Read the model definition and answer for the solid it produces. Units are mm, in the model's axes. A direction names the side the tool comes from. Coordinates: 2 decimals unless noted, no trailing zeros. Loops run counter-clockwise (first coordinate to the right, second up) from the corner with the lowest first, then second, coordinate; pieces in that order, holes last.
Q1. Section D-D (z = 6.25) is taken. Give the vertices of the cut face in (x, y), then the cut area to 3 significant figures.
Q2. Section A-A (x = 0) is taken. Give the vertices of the cut face in (y, z).
Q3. Which of the six approach directions +Z, -Z, +X, -X, +Y, -Y give full straight-line access (tool end or side, diameter ignored) to faces 4 (the face through (0, 0, 5.6)), 5 (the face through (23.846, 7.509, 6.692))?
Q4. Straight lines are drawn through the part: line 1 (Y direction, x = 0, z = 4.5); line 2 (Y direction, x = 0, z = 9.5); line 3 (X direction, y = -0.5, z = 6.5) (3 decimals). For each, find the intervals that lie inside material, in ascending order.
Q5. Flat-ended cylindrical pins translate along their axes: P1, Ø5, axis at x = 8.5, z = 14.5, coming from the +Y side; P2, Ø1.5, axis at x = 19.5, z = 9.5, coming from the +Y side; P3, Ø6, axis at x = 11.5, z = 3.5, coming from the -Y side; P4, Ø10, axis at x = -20, y = 16.5, coming from the -Z side. Find the tip coordinate at first contact, or state that the pin passes through.
Q6. Section C-C (z = 15) is taken. Give the vertices of the cut face in (x, y), then the cut area to 3 significant figures.
Q7. The mould has two halves that part along X. Classify faces 1 (the face through (0, 0, -2)), 2 (the face through (-15, -13, 0)), 3 (the face through (-26.774, 1.178, 6.404)): pulls with the +X half, pulls with the -X half, needs draft (parallel to the pull), parting line crosses it, or undercut.
from build123d import *


with BuildPart() as part:
    # Sketch → Revolution (revolve)
    with BuildSketch(Plane.XZ):
        with BuildLine():
            Line((0, 5.6), (2.5, 5.6))
            Line((2.5, 5.6), (2.5, 2.6))
            Line((2.5, 2.6), (20.5, 2.6))
            Line((20.5, 2.6), (19.5, 0))
            Line((19.5, 0), (25, 0))
            Line((25, 0), (25, 13.2))
            ThreePointArc((25, 13.2), (24.598076, 14.7), (23.5, 15.798076))
            ThreePointArc((24.400016, 17.356913), (23.170591, 17.027501), (23.5, 15.798076))
            ThreePointArc((26.8, 13.2), (26.156926, 15.599992), (24.400016, 17.356913))
            Line((26.8, -0.585786), (26.8, 13.2))
            Line((25.385786, -2), (26.8, -0.585786))
            Line((0, -2), (25.385786, -2))
            Line((0, 5.6), (0, -2))
        make_face()
    revolve(axis=Axis((0, 0, 0), (0, 0, 1)))


solid = part.part
Numbers:
1. outline: circle Ø53.6 at (0, 0); hole circle Ø50 at (0, 0)
1. area: 293 mm2
2. outline: (-26.8, -0.59) - (-25.39, -2) - (25.39, -2) - (26.8, -0.59) - (26.8, 13.2) arc R4.8 ccw to (24.4, 17.36) arc R0.9 ccw to (23.5, 15.8) arc R3 cw to (25, 13.2) - (25, 0) - (19.5, 0) - (20.5, 2.6) - (2.5, 2.6) - (2.5, 5.6) - (-2.5, 5.6) - (-2.5, 2.6) - (-20.5, 2.6) - (-19.5, 0) - (-25, 0) - (-25, 13.2) arc R3 cw to (-23.5, 15.8) arc R0.9 ccw to (-24.4, 17.36) arc R4.8 ccw to (-26.8, 13.2) - close
3. face 4: +Z
3. face 5: none
4. line 1: y = -26.8 to -25, -2.5 to 2.5, 25 to 26.8
4. line 2: y = -26.8 to -25, 25 to 26.8
4. line 3: x = -26.795 to -24.995, 24.995 to 26.795
5. P1: stops at y = 26.06
5. P2: stops at y = 19.15
5. P3: stops at y = -25.42
5. P4: stops at z = -2
6. outline: circle Ø52.9 at (0, 0); hole circle Ø48.8 at (0, 0)
6. area: 327 mm2
7. face 1: needs draft
7. face 2: undercut
7. face 3: parting line crosses it
